Model file for the job. Use its own axes, mm. Face numbers are marked on the shaded views. A direction names the side the tool comes from. Give positions to 0.01 mm unless a question says otherwise; leave off trailing zeros. Loops run counter-clockwise (first coordinate to the right, second up) from the corner with the lowest first, then second, coordinate; pieces in that order, holes last. Notation, with made-up numbers: M 69,39.25 L 109,39.25 A16 cw 109,61.25 Z; hole C 33,7 d1. An arc over 180 degrees is marked long. Answer in a Markdown table with one row per item.
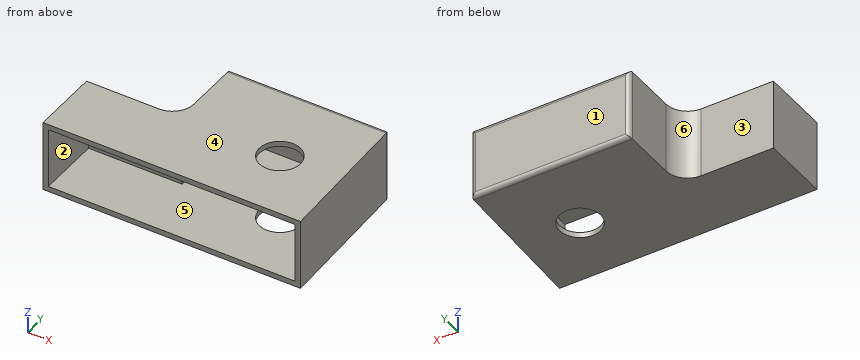
```python
from build123d import *

# Parameters (mm, degrees)
F1_DEPTH = 33.0095589161
F3_R     = 2
F4_T     = -2.5
F5_R     = 10
F2_R     = 9.5732270721
F6_DEPTH = 66.1102235317


with BuildPart() as f1:
    # F0 (on Top) → F1 (new body)
    with BuildSketch(Plane.XY):
        Polygon((62.8429502249, -41.3544625044), (60.3725537658, 27.2316709161), (-13.5185569525, 27.2316709161), (-13.5185569525, -9.4249695539), (-57.1811795235, -9.4249695539), (-57.1811795235, -41.3544625044), align=None)
    extrude(amount=F1_DEPTH)

    # F3
    f3_edges = [f1.edges().sort_by_distance(p)[0] for p in [
        (60.372554, 27.231671, 16.504779),
        (-13.518557, 27.231671, 16.504779),
        (23.426998, 27.231671, 0),
        (23.426998, 27.231671, 33.009559),
    ]]
    fillet(f3_edges, radius=F3_R)

    # F4
    f4_openings = [f1.faces().sort_by_distance(p)[0] for p in [
        (2.830885, -41.354463, 16.504779),
    ]]
    offset(amount=F4_T, openings=f4_openings, kind=Kind.INTERSECTION)

    # F5
    f5_edges = [f1.edges().sort_by_distance(p)[0] for p in [
        (-13.518557, -9.42497, 16.504779),
    ]]
    fillet(f5_edges, radius=F5_R)

    # F2 (on face) → F6 (cut)
    with BuildSketch(Plane.XY.offset(33.0095589161)):
        with Locations((33.1206843257, -9.747531265)):
            Circle(F2_R)
    extrude(amount=-F6_DEPTH, mode=Mode.SUBTRACT)


solid = f1.part
```
Q1. 3-axis set-ups, long thin cutter, end or side, ignore diameter. For the marked faces 1, 2 and 3: which of +Z, -Z, +X, -X, +Y, -Y reach the whole face in a straight line?
Reported:
| item | result |
|---|---|
| face 1 | +Z, -Z, +X, -X, +Y |
| face 2 | -Y |
| face 3 | +Z, -Z, -X, +Y |
Q2. Saw through at B-B (z = 22). Give the cut face in (x, y), and give its area (3 significant figures).
Reported:
| item | result |
|---|---|
| outline | M -57.18,-41.35 L -54.68,-41.35 L -54.68,-11.92 L -11.02,-11.92 L -11.02,24.73 L 57.96,24.73 L 60.34,-41.35 L 62.84,-41.35 L 60.44,25.3 A2 ccw 58.44,27.23 L -11.52,27.23 A2 ccw -13.52,25.23 L -13.52,0.58 A10 cw -23.52,-9.42 L -57.18,-9.42 Z |
| area | 644 mm² |
Q3. Saw through at C-C (y = 19). Give the cut face in (x, z), and give its area (3 significant figures).
Reported:
| item | result |
|---|---|
| outline | M -13.52,0 L 60.67,0 L 60.67,33.01 L -13.52,33.01 Z; hole M -11.02,2.5 L 58.17,2.5 L 58.17,30.51 L -11.02,30.51 Z |
| area | 511 mm² |
Q4. Mould opens along Z. For the marked faces 4, 5 and 6 say: released by +Z, released by -Z, zero draft, split by the parting line, or undercut.
Reported:
| item | result |
|---|---|
| face 4 | released by +Z |
| face 5 | undercut |
| face 6 | zero draft |
Q5. Saw through at A-A (y = -3.5). Give the cut face in (x, z).
Reported:
| item | result |
|---|---|
| outline | M -14.39,0 L 25.87,0 L 25.87,2.5 L -11.02,2.5 L -11.02,30.51 L 25.87,30.51 L 25.87,33.01 L -14.39,33.01 Z; M 40.37,0 L 61.48,0 L 61.48,33.01 L 40.37,33.01 L 40.37,30.51 L 58.98,30.51 L 58.98,2.5 L 40.37,2.5 Z |
Q6. Probe probe 1 along Z at (x, y) = (25, -37.5); probe 2 along Y at (x, z) = (-27, 17); probe 3 along Y at (x, z) = (23.5, 9.5). List the from-to ranges inside material, lowest first.
Reported:
| item | result |
|---|---|
| probe 1 | 0 to 2.5, 30.51 to 33.01 |
| probe 2 | -11.92 to -9.42 |
| probe 3 | 24.73 to 27.23 |
Q7. Drop flat-ended pins along their axis: pin 1 (14 mm diameter, centred on y = 8, z = 15.5, fed in from +X); pin 2 (1 mm diameter, centred on x = -43.5, z = 3.5, fed in from +Y); pin 3 (8 mm diameter, centred on x = 41, z = 8.5, fed in from -Y). Give the stop position or say it passes through.
Reported:
| item | result |
|---|---|
| pin 1 | x = 61.32 |
| pin 2 | y = -9.42 |
| pin 3 | y = 24.73 |
Q8. Saw through at D-D (x = -15). Give the cut face in (y, z).
Reported:
| item | result |
|---|---|
| outline | M -41.35,0 L -4.66,0 L -4.66,33.01 L -41.35,33.01 L -41.35,30.51 L -11.92,30.51 L -11.92,2.5 L -41.35,2.5 Z |
